Read the model definition and answer for the solid it produces. Units are mm, in the model's axes. Face numbers are marked on the shaded views. A direction names the side the tool comes from. Coordinates: 2 decimals unless noted, no trailing zeros. Loops run counter-clockwise (first coordinate to the right, second up) from the corner with the lowest first, then second, coordinate; pieces in that order, holes last.
Q1. Flat-ended cylindrical pins translate along their axes: P1, Ø4, axis at x = 149.5, z = 45, coming from the -Y side; P2, Ø4, axis at x = 60, y = 47, coming from the -Z side; P3, Ø1, axis at x = 73, z = 53, coming from the -Y side. Find the tip coordinate at first contact, or state that the pin passes through.
Q2. Section D-D (x = 116.5) is taken. Give the vertices of the cut face in (y, z), then the cut area to 3 significant figures.
Q3. Section C-C (x = 24.5) is taken. Give the vertices of the cut face in (y, z).
Q4. Section A-A (z = 0) is taken. Give the vertices of the cut face in (x, y), then the cut area to 3 significant figures.
Q5. Straight lines are drawn through the part: line 1 (Y direction, x = 35, z = 0); line 2 (Y direction, x = 190.5, z = 0); line 3 (Z direction, x = 52.5, y = 21). For each, find the intervals that lie inside material, in ascending order.
Q6. The mould has two halves that part along Y. Classify the marked faces 4 and 5: pulls with the +Y half, pulls with the -Y half, needs draft (parallel to the pull), parting line crosses it, or undercut.
Q7. Which of the six approach directions +Z, -Z, +X, -X, +Y, -Y give full straight-line access (tool end or side, diameter ignored) to the marked faces 1, 2 and 3?
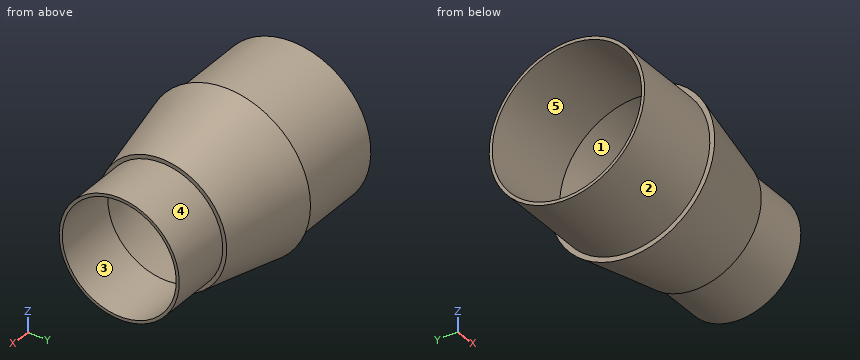
from build123d import *

# Parameters (mm, degrees)
SHELL1_T = -2.54


with BuildPart() as part:
    # Sketch1 → Revolve1 (revolve)
    with BuildSketch(Plane(origin=(0, 0, 0), x_dir=(1, 0, 0), z_dir=(0, 1, 0)), mode=Mode.PRIVATE) as revolve1_sk:
        Polygon((76.2, 68.834), (152.4, 53.34), (152.4, 50.038), (203.2, 50.038), (203.2, 0), (0, 0), (0, 64.77), (76.2, 64.77), align=None)
    revolve(revolve1_sk.sketch.rotate(Axis((0, 0, 0), (1, 0, 0)), 180), axis=Axis((0, 0, 0), (1, 0, 0)))

    # Shell1
    shell1_openings = [part.faces().sort_by_distance(p)[0] for p in [
        (0, 0, 0),
        (203.2, 0, 0),
    ]]
    offset(amount=SHELL1_T, openings=shell1_openings, kind=Kind.INTERSECTION)


solid = part.part
Numbers:
1. P1: stops at y = -32.63
1. P2: stops at z = -46.58
1. P3: stops at y = -37.93
2. outline: circle Ø121.28 at (0, 0); hole circle Ø116.1 at (0, 0)
2. area: 966 mm2
3. outline: circle Ø129.54 at (0, 0); hole circle Ø124.46 at (0, 0)
4. outline: (0, -64.77) - (76.2, -64.77) - (76.2, -68.83) - (152.4, -53.34) - (152.4, -50.04) - (203.2, -50.04) - (203.2, -47.5) - (149.86, -47.5) - (149.86, -51.26) - (78.74, -65.73) - (78.74, -62.23) - (0, -62.23) - close; (0, 62.23) - (78.74, 62.23) - (78.74, 65.73) - (149.86, 51.26) - (149.86, 47.5) - (203.2, 47.5) - (203.2, 50.04) - (152.4, 50.04) - (152.4, 53.34) - (76.2, 68.83) - (76.2, 64.77) - (0, 64.77) - close
4. area: 1,080 mm2
5. line 1: y = -64.77 to -62.23, 62.23 to 64.77
5. line 2: y = -50.04 to -47.5, 47.5 to 50.04
5. line 3: z = -61.27 to -58.58, 58.58 to 61.27
6. face 4: parting line crosses it
6. face 5: undercut
7. face 1: none
7. face 2: -X
7. face 3: +X, -X
